Could you check a few things on this model? Use its own coordinates, in mm. A direction names the side the tool comes from. Coordinates: 2 decimals unless noted, no trailing zeros. Order: outer loops, then holes, each group sorted by start corner. A loop starts at its lowest first (then second) coordinate and runs counter-clockwise, first axis right, second up. Notation, with made-up numbers: (82, 45.5) - (139, 45.5) arc R27 ccw to (139, 62.5) - close; hole circle Ø5 at (-11.75, 25). An arc over 180 degrees is marked (long way). Answer as a JSON object with one key per item and string values. Group by question number.
(1) Will these pins go through, and if not, where does the flat tip stop? P1, Ø8.5, axis at x = -98.5, y = -5, coming from the -Z side; P2, Ø6, axis at x = 14, z = 5, coming from the -Y side.
(2) Which directions (+Z, -Z, +X, -X, +Y, -Y) give clear straight access to the entire face, cutting with the end or side of a thin tool? Please do faces 1 (the flat face through (-2, 0, 0)), 2 (the flat face through (20.14, -4, -20)), 3 (the flat face through (10, -7.62, -5)).
(3) Imagine slicing it at D-D, the plane x = 85.5. Write out the boundary of the cut face in (y, z).
(4) Please list where these lines run through material, in increasing order: probe 1 along X at (y, z) = (-82.5, 6.5); probe 2 along X at (y, z) = (-4.5, -20.5); probe 3 along X at (y, z) = (-84, -16.5).
(5) We'd pull the mould along Z, two halves only. Please class faces 4 (the cylindrical face through (-96.909, -68.146, 26.345)), 5 (the flat face through (56, -7.62, -7)), 6 (the flat face through (-2, -63, 27.94)), 7 (the flat face through (116, -63, -27.94)): pulls with the +Z half, pulls with the -Z half, needs draft (parallel to the pull), parting line crosses it, or undercut.
(6) Imagine slicing it at C-C, the plane z = 10. Write out the boundary of the cut face in (x, y), and give its area (3 significant figures).
(7) Imagine slicing it at B-B, the plane x = -82. Write out the boundary of the cut face in (y, z).
(8) Imagine slicing it at A-A, the plane y = -94.5. Write out the boundary of the cut face in (x, z).
from build123d import *

# Parameters (mm, degrees)
F0_W      = 254
F0_H      = 55.88
F1_DEPTH  = 127
F7_DEPTH  = 251.46
F8_DEPTH  = 251.46
F9_DEPTH  = 251.46
F10_DEPTH = 251.46
F11_DEPTH = 251.46
F12_W     = 18.410387516
F12_H     = 1.8
F12_W_2   = 28.7952162325
F12_W_3   = 28.3505693078
F12_W_4   = 10.2531584787
F13_DEPTH = 28.702
F14_W     = 21.5115528554
F14_H     = 27.94
F14_W_2   = 16.9484987855
F15_DEPTH = 76.2
F17_DEPTH = 7.62


with BuildPart() as f1:
    # F0 (on Front) → F1 (new body)
    with BuildSketch(Plane.XZ):
        Rectangle(F0_W, F0_H)
    extrude(amount=F1_DEPTH)

    # F6 (on face) → F7 (cut)
    with BuildSketch(Plane.XZ.offset(127)):
        with BuildLine():
            ThreePointArc((105.444855988, -27.94), (97.6680144668, 6.3565803399), (89.8911729455, -27.94))
            Line((89.8911729455, -27.94), (105.444855988, -27.94))
        make_face()
    extrude(amount=-F7_DEPTH, mode=Mode.SUBTRACT)

    # F5 (on face) → F8 (cut)
    with BuildSketch(Plane.XZ.offset(127)):
        with BuildLine():
            ThreePointArc((63.3584037423, -27.94), (55.9246577322, 12.700250005), (48.4909117222, -27.94))
            Line((48.4909117222, -27.94), (63.3584037423, -27.94))
        make_face()
    extrude(amount=-F8_DEPTH, mode=Mode.SUBTRACT)

    # F4 (on face) → F9 (cut)
    with BuildSketch(Plane.XZ.offset(127)):
        with BuildLine():
            ThreePointArc((20.1403424144, -27.94), (10.0701712072, 17.5928532036), (0, -27.94))
            Line((0, -27.94), (20.1403424144, -27.94))
        make_face()
    extrude(amount=-F9_DEPTH, mode=Mode.SUBTRACT)

    # F3 (on face) → F10 (cut)
    with BuildSketch(Plane.XZ.offset(127)):
        with BuildLine():
            ThreePointArc((-28.7952162325, -27.94), (-41.4804015309, 21.8266300514), (-54.1655868292, -27.94))
            Line((-54.1655868292, -27.94), (-28.7952162325, -27.94))
        make_face()
    extrude(amount=-F10_DEPTH, mode=Mode.SUBTRACT)

    # F2 (on face) → F11 (cut)
    with BuildSketch(Plane.XZ.offset(127)):
        with BuildLine():
            Line((-107.5928583741, -27.94), (-88.4136334062, -27.94))
            ThreePointArc((-88.4136334062, -27.94), (-98.0032458901, 26.3666404622), (-107.5928583741, -27.94))
        make_face()
    extrude(amount=-F11_DEPTH, mode=Mode.SUBTRACT)

    # F12 (on face) → F13 (cut)
    with BuildSketch(Plane(origin=(0, 0, -27.94), x_dir=(1, 0, 0), z_dir=(0, 0, -1))):
        with Locations((-116.7980521321, 3.44)):
            Rectangle(F12_W, F12_H)
        Polygon((-70.0032458901, 4.34), (-88.4136334062, 4.34), (-88.4136334062, 2.54), (-70.0032458901, 2.54), (-54.1655868292, 2.54), (-54.1655868292, 4.34), align=None)
        with Locations((-14.3976081163, 3.44)):
            Rectangle(F12_W_2, F12_H)
        with Locations((34.3156270683, 3.44)):
            Rectangle(F12_W_3, F12_H)
        Polygon((89.8911729455, 4.34), (63.3584037423, 4.34), (63.3584037423, 2.54), (79.6380144668, 2.54), (89.8911729455, 2.54), align=None)
        with Locations((110.5714352274, 3.44)):
            Rectangle(F12_W_4, F12_H)
    extrude(amount=-F13_DEPTH, mode=Mode.SUBTRACT)

    # F14 (on face) → F15 (cut)
    with BuildSketch(Plane(origin=(0, 0, 0), x_dir=(-1, 0, 0), z_dir=(0, 1, 0))):
        Polygon((-91.1045372486, -21.9016313345), (-104.6037971973, -25.1468683294), (-104.6037971973, -27.94), (-91.1045372486, -27.94), align=None)
        Polygon((-104.6037971973, 0), (-104.6037971973, -25.1468683294), (-91.1045372486, -21.9016313345), (-91.1045372486, 0), align=None)
        with BuildLine():
            Line((-48.8363243639, -11.7403062927), (-63.663393259, -15.3047500242))
            Line((-63.663393259, -15.3047500242), (-63.663393259, -27.8218393414))
            ThreePointArc((-63.663393259, -27.8218393414), (-63.5111285509, -27.8815134631), (-63.3584037423, -27.94))
            Line((-63.3584037423, -27.94), (-48.8363243639, -27.94))
            Line((-48.8363243639, -27.94), (-48.8363243639, -11.7403062927))
        make_face()
        Polygon((-63.663393259, 0), (-63.663393259, -15.3047500242), (-48.8363243639, -11.7403062927), (-48.8363243639, 0), align=None)
        with BuildLine():
            ThreePointArc((-81.4663434771, -19.5845989112), (-101.8823771095, 5.857126467), (-108.5034271854, -26.0843436838))
            Line((-108.5034271854, -26.0843436838), (-104.6037971973, -25.1468683294))
            Line((-104.6037971973, -25.1468683294), (-104.6037971973, 0))
            Line((-104.6037971973, 0), (-91.1045372486, 0))
            Line((-91.1045372486, 0), (-91.1045372486, -21.9016313345))
            Line((-91.1045372486, -21.9016313345), (-81.4663434771, -19.5845989112))
        make_face()
        with Locations((40.9021200612, -13.97)):
            Rectangle(F14_W, F14_H)
        with Locations((99.0267731249, -13.97)):
            Rectangle(F14_W_2, F14_H)
    extrude(amount=-F15_DEPTH, mode=Mode.SUBTRACT)

    # F16 (on face) → F17 (join)
    with BuildSketch(Plane(origin=(0, 0, 0), x_dir=(-1, 0, 0), z_dir=(0, 1, 0))):
        Polygon((127, 27.94), (-127, 27.94), (-127, -27.94), (-105.444855988, -27.94), (-105.444855988, -11.3536855206), (-90.5294641852, -11.3536855206), (-89.8911729455, -27.94), (-63.3584037423, -27.94), (-63.3584037423, -11.3536855206), (-48.4909117222, -11.3536855206), (-48.4909117222, -27.94), (-20.1403424144, -27.94), (-20.1403424144, -11.3536855206), (0, -11.3536855206), (0, -27.94), (28.7952162325, -27.94), (28.7952162325, -11.3536855206), (53.1729161739, -11.3536855206), (54.1655868292, -27.94), (88.4136334062, -27.94), (88.4136334062, -11.3536855206), (107.4278950691, -11.3536855206), (107.5928583741, -27.94), (127, -27.94), align=None)
    extrude(amount=-F17_DEPTH)


solid = f1.part
Result set:
{
 "1": {"P1": "stops at z = -11.35", "P2": "stops at y = -7.62"},
 "2": {"face 1": "+Z, -Z, +X, -X, +Y", "face 2": "-Z, +Y, -Y", "face 3": "-Y"},
 "3": {"outline": "(-127, -27.94) - (0, -27.94) - (0, 27.94) - (-127, 27.94) - (-127, 1.63) - (-7.62, 1.63) - (-7.62, -24.98) - (-127, -24.98) - close"},
 "4": {"probe 1": "x = -127 to -124.8, -71.21 to -65.51, -17.45 to -10.1, 30.24 to 41.03, 70.82 to 127", "probe 2": "x = -127 to -107.52, -88.41 to -53.72, -28.8 to 0, 20.14 to 48.49, 63.36 to 90.18, 105.44 to 127", "probe 3": "x = -127 to -121.73, -74.28 to -65.19, -17.77 to -11.52, 31.66 to 36.59, 75.26 to 80.3, 115.04 to 127"},
 "5": {"face 4": "undercut", "face 5": "undercut", "face 6": "pulls with the +Z half", "face 7": "pulls with the -Z half"},
 "6": {"outline": "(-127, -127) - (-123.47, -127) - (-123.47, -7.62) - (-72.53, -7.62) - (-72.53, -127) - (-63.55, -127) - (-63.55, -7.62) - (-19.41, -7.62) - (-19.41, -127) - (-7.39, -127) - (-7.39, -7.62) - (27.53, -7.62) - (27.53, -127) - (45.62, -127) - (45.62, -7.62) - (66.23, -7.62) - (66.23, -127) - (127, -127) - (127, 0) - (-127, 0) - close", "area": "14,300 mm^2"},
 "7": {"outline": "(-127, -27.94) - (0, -27.94) - (0, 27.94) - (-127, 27.94) - (-127, 21.34) - (-7.62, 21.34) - (-7.62, -24.61) - (-127, -24.61) - close"},
 "8": {"outline": "(-127, -27.94) - (-107.59, -27.94) arc R28 cw (long way) to (-88.41, -27.94) - (-54.17, -27.94) arc R26.5 cw (long way) to (-28.8, -27.94) - (0, -27.94) arc R23.88 cw (long way) to (20.14, -27.94) - (48.49, -27.94) arc R21 cw (long way) to (63.36, -27.94) - (89.89, -27.94) arc R18.03 cw (long way) to (105.44, -27.94) - (127, -27.94) - (127, 27.94) - (-127, 27.94) - close"}
}
